The drawing under review shows one solid part. Ordinate dimensions are in mm from its lowest x, y, z. A direction names the side the tool comes from. Coordinates: 2 decimals unless noted, no trailing zeros. Order: outer loops, then holes, each group sorted by start corner. A loop starts at its lowest first (then second) coordinate and runs counter-clockwise, first axis right, second up. Notation, with made-up numbers: (-37, 77) - (20, 77) arc R17 ccw to (20, 110) - close; hole circle Ø4 at (40, -14). An arc over 180 degrees is marked (long way). Write each question's results on one line, items separated by ' | '. Start each with the question number.
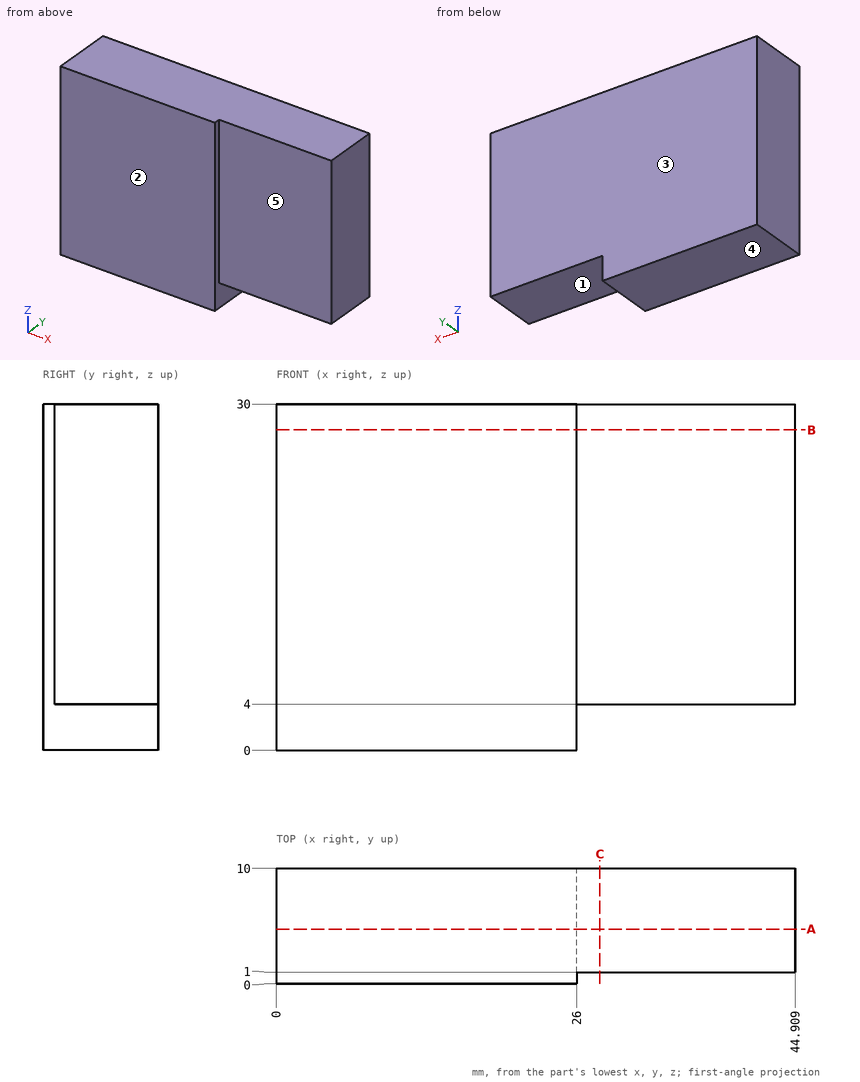
(1) To check wall thickness, follow line 1 along Y through (x, z) = (33.5, 11.75); line 2 along Z through (x, y) = (27.5, 3.25); line 3 along X through (y, z) = (1.5, 1.75). State the ranges of each line that lie inside material, in increasing order. Write a range as [from, to].
(2) Clearance check with a flat-ended pin moving along its axis: pin 1 (15 mm diameter, centred on x = 37, z = 21, fed in from -Y). State where the tip first meets the part, or that it passes through.
(3) Take a section at A-A (y = 4.75). State the section outline as (x, z) points, plus the area to 3 significant figures.
(4) Mouldability with a two-part tool opening along Y and no side actions: class the marked faces 3, 4 and 5 as +Y half, -Y half, draft (parallel to the pull), parting line (faces both ways), or undercut.
(5) Tool access review of the marked faces 1 and 2: name each direction out of +Z, -Z, +X, -X, +Y, -Y from which nothing blocks a thin tool from reaching the whole face with its end or side.
(6) Take a section at B-B (z = 27.75). State the section outline as (x, y) points, plus the area to 3 significant figures.
(7) Take a section at C-C (x = 28). State the section outline as (y, z) points, plus the area to 3 significant figures.
Worked out:
1) line 1: [1, 10] | line 2: [4, 30] | line 3: [0, 26]
2) pin 1: y = 1
3) outline: (0, 0) - (26, 0) - (26, 4) - (44.91, 4) - (44.91, 30) - (0, 30) - close | area: 1,270 mm^2
4) face 3: +Y half | face 4: draft | face 5: -Y half
5) face 1: -Z, +X, +Y, -Y | face 2: +Z, -Z, +X, -X, -Y
6) outline: (0, 0) - (26, 0) - (26, 1) - (44.91, 1) - (44.91, 10) - (0, 10) - close | area: 430 mm^2
7) outline: (1, 4) - (10, 4) - (10, 30) - (1, 30) - close | area: 234 mm^2
